```python
from build123d import *

# Parameters (mm, degrees)
PAD020_DEPTH  = 30
SKETCH004_R   = 3
HOLE003_DEPTH = 46.001
FILLET_R      = 14
FILLET011_R   = 3
FILLET012_R   = 2


with BuildPart() as part:
    # Sketch036 → Pad020 (new body)
    with BuildSketch(Plane.YZ):
        Polygon((-23, 50), (-21, 50), (-21, 2), (21, 2), (21, 50), (23, 50), (23, 0), (-23, 0), align=None)
    extrude(amount=PAD020_DEPTH)

    # Sketch004 (on Face8 of Pad020) → Hole003 (cut, through all)
    with BuildSketch(Plane(origin=(0, -23, 0), x_dir=(0, 0, -1), z_dir=(0, -1, 0))):
        with Locations((-35, 15)):
            Circle(SKETCH004_R)
    extrude(amount=-HOLE003_DEPTH, mode=Mode.SUBTRACT)

    # Fillet
    fillet_edges = [part.edges().sort_by_distance(p)[0] for p in [
        (30, 22, 50),
        (30, -22, 50),
        (0, -22, 50),
        (0, 22, 50),
    ]]
    fillet(fillet_edges, radius=FILLET_R)

    # Fillet011
    fillet011_edges = [part.edges().sort_by_distance(p)[0] for p in [
        (15, 21, 2),
        (15, -21, 2),
    ]]
    fillet(fillet011_edges, radius=FILLET011_R)

    # Fillet012
    fillet012_edges = [part.edges().sort_by_distance(p)[0] for p in [
        (15, -23, 0),
        (15, 23, 0),
    ]]
    fillet(fillet012_edges, radius=FILLET012_R)


solid = part.part
```
Here's how the part is built. I have some questions about the finished solid (model axes, mm). A direction names the side the tool comes from. Coordinates: 2 decimals unless noted, no trailing zeros. Write each loop counter-clockwise with the first axis right and the second up, starting at its lowest first coordinate (ties: lowest second). Pieces come first, ordered by that corner, then holes. Notation, with made-up numbers: (-13.75, 52.5) - (20.25, 52.5) arc R23 cw to (20.25, 84.5) - close; hole circle Ø2 at (44, 8.5). An arc over 180 degrees is marked (long way). One line per item, written item: value.
1) On a 3-axis mill with a long thin cutter (end or side, diameter ignored), from which of +Z, -Z, +X, -X, +Y, -Y can I reach the whole of each face in a straight line? I mean faces 4 (the flat face through (15, 0, 2)), 5 (the cylindrical face through (26, 22, 45.8)). Say none if no direction works.
Model answer:
face 4: +Z, +X, -X
face 5: +Z, +X, +Y, -Y
2) I need wall thicknesses on line 1 along Y through (x, z) = (9.5, 35.5); line 2 along X through (y, z) = (22, 35); line 3 along Z through (x, y) = (15, 9.5). Which ranges of each line are inside material? Lowest first, please.
Model answer:
line 1: y = -23 to -21, 21 to 23
line 2: x = 0 to 12, 18 to 30
line 3: z = 0 to 2
3) Suppose I cut it at D-D on y = 13. Write out the boundary of the cut face in (x, z), and give its area (3 significant figures).
Model answer:
outline: (0, 0) - (30, 0) - (30, 2) - (0, 2) - close
area: 60.0 mm²
4) Suppose I cut it at A-A on z = 15. Write out the boundary of the cut face in (x, y).
Model answer:
outline: (0, -23) - (30, -23) - (30, -21) - (0, -21) - close; (0, 21) - (30, 21) - (30, 23) - (0, 23) - close
5) Suppose I cut it at C-C on z = 35. Write out the boundary of the cut face in (x, y).
Model answer:
outline: (0, -23) - (12, -23) - (12, -21) - (0, -21) - close; (0, 21) - (12, 21) - (12, 23) - (0, 23) - close; (18, -23) - (30, -23) - (30, -21) - (18, -21) - close; (18, 21) - (30, 21) - (30, 23) - (18, 23) - close
6) We'd pull the mould along Y, two halves only. Please class faces 1 (the cylindrical face through (15.21, -20.14, 2.9)), 2 (the flat face through (15, 0, 0)), 3 (the flat face through (15, 23, 26)): pulls with the +Y half, pulls with the -Y half, needs draft (parallel to the pull), parting line crosses it, or undercut.
Model answer:
face 1: undercut
face 2: needs draft
face 3: pulls with the +Y half
7) Suppose I cut it at B-B on x = 15. Write out the boundary of the cut face in (y, z).
Model answer:
outline: (-23, 2) arc R2 ccw to (-21, 0) - (21, 0) arc R2 ccw to (23, 2) - (23, 32) - (21, 32) - (21, 5) arc R3 cw to (18, 2) - (-18, 2) arc R3 cw to (-21, 5) - (-21, 32) - (-23, 32) - close; (-23, 38) - (-21, 38) - (-21, 50) - (-23, 50) - close; (21, 38) - (23, 38) - (23, 50) - (21, 50) - close
